```python
from build123d import *

# Parameters (mm, degrees)
F1_DEPTH  = 3
F2_R      = 1.5
F2_R_2    = 2
F3_DEPTH  = 5
F4_R      = 1.5
F4_R_2    = 2
F5_DEPTH  = 5
F6_W      = 5
F6_H      = 8
F7_DEPTH  = 20
F9_DEPTH  = 25.4
F10_R     = 2
F11_DEPTH = 25.4
F12_W     = 20
F12_H     = 20
F13_DEPTH = 7.5
F14_R     = 1.7
F15_DEPTH = 5
F16_DEPTH = 15
F18_DEPTH = 10


with BuildPart() as f1:
    # F0 (on Top) → F1 (new body)
    with BuildSketch(Plane.XY):
        Polygon((-50, -18.5), (50, -18.5), (50, 18.5), (75, 18.5), (75, 76.5), (-75, 76.5), (-75, 18.5), (-50, 18.5), align=None)
    extrude(amount=-F1_DEPTH)

    # F2 (on face) → F3 (join)
    with BuildSketch(Plane.YZ.offset(75)):
        with BuildLine():
            Line((18.5, 10), (18.5, -3))
            Line((18.5, -3), (64.5, -3))
            Line((64.5, -3), (64.5, 10))
            ThreePointArc((64.5, 10), (61.5710678119, 17.0710678119), (54.5, 20))
            Line((54.5, 20), (28.5, 20))
            ThreePointArc((28.5, 20), (21.4289321881, 17.0710678119), (18.5, 10))
        make_face()
        with Locations((22.5, 13)):
            Circle(F2_R, mode=Mode.SUBTRACT)
        with Locations((60.5, 13)):
            Circle(F2_R, mode=Mode.SUBTRACT)
        with Locations((41.5, 17)):
            Circle(F2_R_2, mode=Mode.SUBTRACT)
    extrude(amount=-F3_DEPTH)

    # F4 (on face) → F5 (join)
    with BuildSketch(Plane(origin=(-75, 0, 0), x_dir=(0, -1, 0), z_dir=(-1, 0, 0))):
        with BuildLine():
            Line((-64.5, 10), (-64.5, 0))
            Line((-64.5, 0), (-18.5, 0))
            Line((-18.5, 0), (-18.5, 10))
            ThreePointArc((-18.5, 10), (-21.4289321881, 17.0710678119), (-28.5, 20))
            Line((-28.5, 20), (-54.5, 20))
            ThreePointArc((-54.5, 20), (-61.5710678119, 17.0710678119), (-64.5, 10))
        make_face()
        with Locations((-60.5, 13)):
            Circle(F4_R, mode=Mode.SUBTRACT)
        with Locations((-22.5, 13)):
            Circle(F4_R, mode=Mode.SUBTRACT)
        with Locations((-41.5, 17)):
            Circle(F4_R_2, mode=Mode.SUBTRACT)
    extrude(amount=-F5_DEPTH)

    # F6 (on face) → F7 (join)
    with BuildSketch(Plane.XY):
        with Locations((-29.5, 41.5)):
            Rectangle(F6_W, F6_H)
        with Locations((-29.5, 17.5)):
            Rectangle(F6_W, F6_H)
        with Locations((-29.5, -6.5)):
            Rectangle(F6_W, F6_H)
        with Locations((-12.5, 41.5)):
            Rectangle(F6_W, F6_H)
        with Locations((-12.5, -6.5)):
            Rectangle(F6_W, F6_H)
    extrude(amount=F7_DEPTH)

    # F8 (on face) → F9 (cut)
    with BuildSketch(Plane(origin=(-32, 0, 0), x_dir=(0, -1, 0), z_dir=(-1, 0, 0))):
        with BuildLine():
            Line((4.48324112, 22.2221616161), (4.5000102861, 16.9935856035))
            ThreePointArc((4.5000102861, 16.9935856035), (6.5287446527, 15.0002065744), (8.4993478236, 17.0510713252))
            Line((8.4993478236, 17.0510713252), (8.3693183096, 22.1414860464))
            Line((8.3693183096, 22.1414860464), (4.48324112, 22.2221616161))
        make_face()
        with BuildLine():
            Line((-19.5, 20.0955439359), (-19.5, 17))
            ThreePointArc((-19.5, 17), (-17.5, 15), (-15.5, 17))
            Line((-15.5, 17), (-15.5, 20.6426493824))
            Line((-15.5, 20.6426493824), (-19.5, 20.0955439359))
        make_face()
    extrude(amount=-F9_DEPTH, mode=Mode.SUBTRACT)

    # F10 (on face) → F11 (cut)
    with BuildSketch(Plane(origin=(-32, 0, 0), x_dir=(0, -1, 0), z_dir=(-1, 0, 0))):
        with Locations((-41.5, 17)):
            Circle(F10_R)
    extrude(amount=-F11_DEPTH, mode=Mode.SUBTRACT)

    # F12 (on face) → F13 (join)
    with BuildSketch(Plane.XY):
        with Locations((19, 17.5)):
            Rectangle(F12_W, F12_H)
    extrude(amount=F13_DEPTH)

    # F14 (on face) → F15 (cut)
    with BuildSketch(Plane(origin=(9, 0, 0), x_dir=(0, -1, 0), z_dir=(-1, 0, 0))):
        Polygon((-22.5, -1.079571669), (-19.4, 0.7102141655), (-19.4, 4.2897858345), (-25.6, 4.2897858345), (-25.6, 0.7102141655), align=None)
        with Locations((-22.5, 2.5)):
            Circle(F14_R, mode=Mode.SUBTRACT)
        Polygon((-25.6, 4.2897858345), (-19.4, 4.2897858345), (-22.5, 6.079571669), align=None)
        Polygon((-22.5, 6.079571669), (-19.4, 4.2897858345), (-19.4, 10.6374248862), (-25.6, 10.6374248862), (-25.6, 4.2897858345), align=None)
        Polygon((-12.5, -1.079571669), (-9.4, 0.7102141655), (-9.4, 4.2897858345), (-15.6, 4.2897858345), (-15.6, 0.7102141655), align=None)
        with Locations((-12.5, 2.5)):
            Circle(F14_R, mode=Mode.SUBTRACT)
        Polygon((-15.6, 4.2897858345), (-9.4, 4.2897858345), (-12.5, 6.079571669), align=None)
        Polygon((-12.5, 6.079571669), (-9.4, 4.2897858345), (-9.3752695248, 4.2897858345), (-9.3752695248, 11.5191247314), (-15.6, 11.5191247314), (-15.6, 4.2897858345), align=None)
        with Locations((-22.5, 2.5)):
            Circle(F14_R)
        with Locations((-12.5, 2.5)):
            Circle(F14_R)
    extrude(amount=-F15_DEPTH, mode=Mode.SUBTRACT)

    # F14 (on face) → F16 (cut)
    with BuildSketch(Plane(origin=(9, 0, 0), x_dir=(0, -1, 0), z_dir=(-1, 0, 0))):
        with Locations((-22.5, 2.5)):
            Circle(F14_R)
        with Locations((-12.5, 2.5)):
            Circle(F14_R)
    extrude(amount=-F16_DEPTH, mode=Mode.SUBTRACT)

    # F17 (on face) → F18 (cut)
    with BuildSketch(Plane(origin=(14, 0, 0), x_dir=(0, -1, 0), z_dir=(-1, 0, 0))):
        with BuildLine():
            Line((-14.2, 7.5), (-14.2, 2.5))
            ThreePointArc((-14.2, 2.5), (-12.5, 4.2), (-10.8, 2.5))
            Line((-10.8, 2.5), (-10.8, 7.5))
            Line((-10.8, 7.5), (-14.2, 7.5))
        make_face()
    extrude(amount=-F18_DEPTH, mode=Mode.SUBTRACT)


solid = f1.part
```
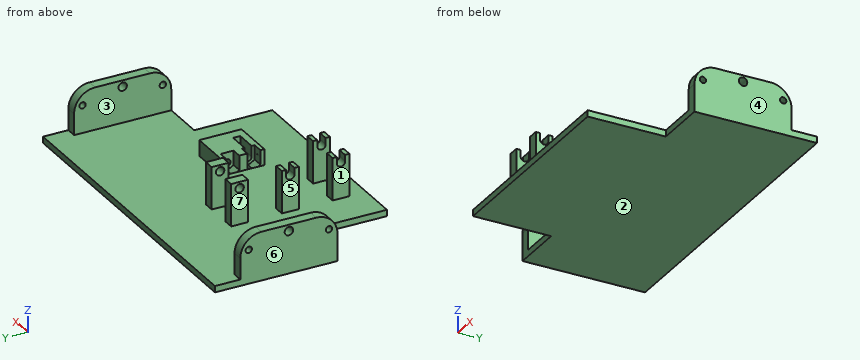
Can you work these out from the model? Positions are in its coordinate system, mm. Face numbers are marked on the shaded views. A direction names the side the tool comes from. Give positions to 0.01 mm unless a question says otherwise; leave off trailing zeros. Write each loop counter-clockwise with the first axis right and the second up, starting at its lowest first coordinate (ties: lowest second). Pieces come first, ordered by that corner, then holes. Notation, with made-up numbers: (-28.75, 56.25) -> (-0.75, 56.25) arc R24 cw to (-0.75, 85.25) -> close; hole circle Ø6 at (16.25, 57.25). An arc over 180 degrees is marked (long way). One line per item, written item: value.
Q1. Imagine slicing it at A-A on y = 41.5. Give the number of separate pieces and of enclosed holes in the cut face, and give its area (3 significant figures).
Results found:
separate pieces: 5
enclosed holes: 0
area: 770 mm^2
Q2. We'd pull the mould along X, two halves only. Please class the marked faces 4, 5, 6 and 7: +X half, -X half, draft (parallel to the pull), parting line (faces both ways), or undercut.
Results found:
face 4: +X half
face 5: undercut
face 6: -X half
face 7: undercut
Q3. Please list where these lines run through material, in increasing order: line 1 (X direction, y = 24, z = 3.75); line 2 (X direction, y = 27, z = 6.5); line 3 (X direction, y = 40.5, z = 13). Write a range as [from, to].
Results found:
line 1: x = [-75, -70], [14, 29], [70, 75]
line 2: x = [-75, -70], [9, 29], [70, 75]
line 3: x = [-75, -70], [-32, -27], [-15, -10], [70, 75]
Q4. For P1, Ø5, axis at x = 17.5, y = 65, coming from the +Z side; P2, Ø0.9, axis at y = 8.5, z = 2, coming from the -X side; P3, Ø4, axis at x = 20, z = 5.5, coming from the +Y side; P4, Ø12, axis at x = 58, y = -7.5, coming from the +Z side, each with a flat end and sliding along its axis, tell me the tip position at first contact or that it passes through.
Results found:
P1: stops at z = 0
P2: stops at x = 9
P3: stops at y = 27.5
P4: passes through
Q5. Imagine slicing it at D-D on y = 3. Please give me the cut outline in (x, z), and give its area (3 significant figures).
Results found:
outline: (-50, -3) -> (50, -3) -> (50, 0) -> (-50, 0) -> close
area: 300 mm^2
Q6. Imagine slicing it at B-B on y = -6.5. Please give me the cut outline in (x, z).
Results found:
outline: (-50, -3) -> (50, -3) -> (50, 0) -> (-10, 0) -> (-10, 15) -> (-15, 15) -> (-15, 0) -> (-27, 0) -> (-27, 15) -> (-32, 15) -> (-32, 0) -> (-50, 0) -> close
Q7. Imagine slicing it at C-C on x = 62.5. Please give me the cut outline in (y, z).
Results found:
outline: (18.5, -3) -> (76.5, -3) -> (76.5, 0) -> (18.5, 0) -> close
Q8. Which directions (+Z, -Z, +X, -X, +Y, -Y) give clear straight access to the entire face, cutting with the end or side of a thin tool? Please do the marked faces 1, 2 and 3.
Results found:
face 1: +Z, -X, +Y, -Y
face 2: -Z, +X, -X, +Y, -Y
face 3: +Z, +Y, -Y
